Autodesk Fusion 360 part; units mm, degrees
sketch "Sketch1" plane through (0, 0, 0) normal (0, 1, 0) x (1, 0, 0) in component "Base Plate"
  line L0 (-125, 50) -> (125, 50)
  line L1 (125, 50) -> (125, -50)
  line L2 (125, -50) -> (-125, -50)
  line L3 (-125, -50) -> (-125, 50)
  line L4 (-125, 50) -> (125, -50) construction
  line L5 (125, 50) -> (-125, -50) construction
  circle A0 centre (-110, 35) radius 6
  circle A1 centre (-110, -35) radius 6
  line L6 (0, 0) -> (0, 50) construction
  circle A2 centre (110, 35) radius 6
  circle A3 centre (110, -35) radius 6
  dimension "d1" = 100
  dimension "d2" = 250
  dimension "d3" = 15
  dimension "d4" = 15
  dimension "d5" = 12
  dimension "d6" = 15
extrude "Extrude1" add sketch "Sketch1" against normal blind 10 in component "Base Plate"
component "Base Plate" placed x (1, 0, 0) y (0, 1, 0) z (0, 0, 1) at (0, 0, 0)
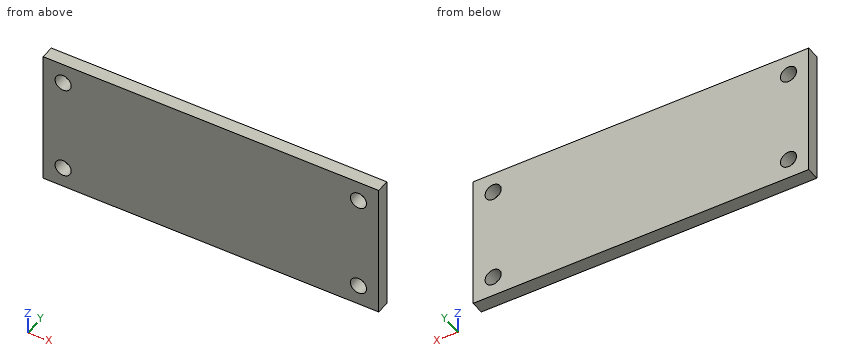
CAD build for the part. Positions are in the model's coordinates, mm. Round coordinates to 2 decimals unless told otherwise and drop trailing zeros. Write each loop counter-clockwise with the first axis right and the second up, starting at its lowest first coordinate (ties: lowest second). Pieces come first, ordered by that corner, then holes. Notation, with made-up numbers: (17, -27) - (30, -27) arc R29 cw to (30, -1) - close; hole circle Ø8 at (-40, 85.5). An arc over 180 degrees is marked (long way). Write item = value, one per line. Start each with the question number.
Q1. Band-saw the part on C-C (z = -35). Give the cut face in (x, y), then the cut area to 3 significant figures.
Q2. Band-saw the part on A-A (x = 110). Give the cut face in (y, z).
Q3. Probe L1, parallel to X at y = -2.75, z = -35; L2, parallel to Z at x = -110, y = -1.75; L3, parallel to X at y = -6, z = 36. List the from-to ranges inside material, lowest first. Write a range as from..to.
Q4. Band-saw the part on B-B (y = -7). Give the cut face in (x, z), then the cut area to 3 significant figures.
Answers below:
q1.outline = (-125, -10) - (-116, -10) - (-116, 0) - (-125, 0) - close; (-104, -10) - (104, -10) - (104, 0) - (-104, 0) - close; (116, -10) - (125, -10) - (125, 0) - (116, 0) - close
q1.area = 2,260 mm2
q2.outline = (-10, -50) - (0, -50) - (0, -41) - (-10, -41) - close; (-10, -29) - (0, -29) - (0, 29) - (-10, 29) - close; (-10, 41) - (0, 41) - (0, 50) - (-10, 50) - close
q3.L1 = -125..-116, -104..104, 116..125
q3.L2 = -50..-41, -29..29, 41..50
q3.L3 = -125..-115.92, -104.08..104.08, 115.92..125
q4.outline = (-125, -50) - (125, -50) - (125, 50) - (-125, 50) - close; hole circle Ø12 at (-110, -35); hole circle Ø12 at (-110, 35); hole circle Ø12 at (110, -35); hole circle Ø12 at (110, 35)
q4.area = 24,500 mm2
